from build123d import *

# Parameters (mm, degrees)
SKETCH1_R             = 40
BOSS_EXTRUDE1_DEPTH   = 105
SKETCH2_R             = 25
BOSS_EXTRUDE2_DEPTH   = 21
BOSS_EXTRUDE3_START   = 21
SKETCH3_R             = 25
BOSS_EXTRUDE3_DEPTH   = 21
FILLET1_R             = 2
SKETCH5_W             = 45.050033199
SKETCH5_H             = 42.615736352
CUT_EXTRUDE1_DEPTH    = 158.508729917
CUT_EXTRUDE2_DEPTH    = 158.508729917
SKETCH8_R             = 3.75
CUT_EXTRUDE3_DEPTH    = 158.508729917
CUT_EXTRUDE4_DEPTH    = 139.115893365
CUT_EXTRUDE5_DEPTH    = 10
FILLET2_R             = 1
BODY_MOVE_COPY1_ANGLE = 90


with BuildPart() as part:
    # Sketch1 → Boss-Extrude1 (new body)
    with BuildSketch(Plane(origin=(0, 0, 0), x_dir=(1, 0, 0), z_dir=(0, 1, 0))):
        with Locations(Location((0, 0, 0), (0, 0, 270))):
            Circle(SKETCH1_R)
    extrude(amount=BOSS_EXTRUDE1_DEPTH)

    # Sketch2 → Boss-Extrude2 (add)
    with BuildSketch(Plane(origin=(0, 105, 0), x_dir=(1, 0, 0), z_dir=(0, 1, 0))):
        with Locations(Location((0, 0, 0), (0, 0, 90))):
            Circle(SKETCH2_R)
    extrude(amount=BOSS_EXTRUDE2_DEPTH)

    # Sketch3 → Boss-Extrude3 (add)
    with BuildSketch(Plane(origin=(0, 0, 0), x_dir=(-1, 0, 0), z_dir=(0, -1, 0)).offset(BOSS_EXTRUDE3_START)):
        with Locations(Location((0, 0, 0), (0, 0, 90))):
            Circle(SKETCH3_R)
    extrude(amount=-BOSS_EXTRUDE3_DEPTH)

    # Fillet1
    fillet1_edges = [part.edges().sort_by_distance(p)[0] for p in [
        (0, 0, 25),
        (0, 105, 25),
    ]]
    fillet(fillet1_edges, radius=FILLET1_R)

    # Sketch4 → Cut-Revolve1 (revolve, cut)
    with BuildSketch(Plane(origin=(0, 0, 0), x_dir=(0, 0, -1), z_dir=(1, 0, 0)), mode=Mode.PRIVATE) as cut_revolve1_sk:
        Polygon((40, 73.5), (37.5, 71), (37.5, 34), (40, 31.5), align=None)
    revolve(cut_revolve1_sk.sketch.rotate(Axis((0, 105, 0), (0, -1, 0)), 180), axis=Axis((0, 105, 0), (0, -1, 0)), mode=Mode.SUBTRACT)

    # Sketch5 → Cut-Extrude1 (cut, through all)
    with BuildSketch(Plane(origin=(0, -21, 0), x_dir=(-1, 0, 0), z_dir=(0, -1, 0))):
        with Locations((-22.5250166, -21.307868176)):
            Rectangle(SKETCH5_W, SKETCH5_H)
    extrude(amount=-CUT_EXTRUDE1_DEPTH, mode=Mode.SUBTRACT)

    # Sketch7 → Cut-Extrude2 (cut, through all)
    with BuildSketch(Plane(origin=(0, -21, 0), x_dir=(-1, 0, 0), z_dir=(0, -1, 0))):
        with BuildLine():
            Line((12, -13), (-12, -13))
            ThreePointArc((-12, -13), (-15, -10), (-12, -7))
            Line((-12, -7), (12, -7))
            ThreePointArc((12, -7), (15, -10), (12, -13))
        make_face()
    extrude(amount=-CUT_EXTRUDE2_DEPTH, mode=Mode.SUBTRACT)

    # Sketch8 → Cut-Extrude3 (cut, through all)
    with BuildSketch(Plane(origin=(0, -21, 0), x_dir=(-1, 0, 0), z_dir=(0, -1, 0))):
        with Locations(Location((8.282209443, -30.909626441, 0), (0, 0, 270))):
            Circle(SKETCH8_R)
        with Locations((-8.282209443, -30.909626441)):
            Circle(SKETCH8_R)
        with Locations((-22.627416998, -22.627416998)):
            Circle(SKETCH8_R)
        with Locations((-30.909626441, -8.282209443)):
            Circle(SKETCH8_R)
        with Locations(Location((-30.909626441, 8.282209443, 0), (0, 0, 270))):
            Circle(SKETCH8_R)
        with Locations(Location((-22.627416998, 22.627416998, 0), (0, 0, 270))):
            Circle(SKETCH8_R)
        with Locations(Location((-8.282209443, 30.909626441, 0), (0, 0, 270))):
            Circle(SKETCH8_R)
        with Locations(Location((8.282209443, 30.909626441, 0), (0, 0, 270))):
            Circle(SKETCH8_R)
        with Locations(Location((22.627416998, 22.627416998, 0), (0, 0, 270))):
            Circle(SKETCH8_R)
        with Locations(Location((30.909626441, 8.282209443, 0), (0, 0, 270))):
            Circle(SKETCH8_R)
        with Locations(Location((30.909626441, -8.282209443, 0), (0, 0, 270))):
            Circle(SKETCH8_R)
        with Locations(Location((22.627416998, -22.627416998, 0), (0, 0, 270))):
            Circle(SKETCH8_R)
    extrude(amount=-CUT_EXTRUDE3_DEPTH, mode=Mode.SUBTRACT)

    # Sketch9 → Cut-Extrude4 (cut, through all)
    with BuildSketch(Plane.XY):
        with BuildLine():
            Line((25, 123.355095289), (40, 126))
            Line((40, 126), (30.207539179, 105))
            Line((30.207539179, 105), (40, 105))
            Line((40, 105), (40, 96))
            ThreePointArc((40, 96), (61.213203436, 104.786796564), (70, 126))
            ThreePointArc((70, 126), (40, 156), (10, 126))
            Line((10, 126), (25, 126))
            Line((25, 126), (25, 123.355095289))
        make_face()
        with BuildLine():
            Line((30.207539179, 105), (40, 126))
            Line((40, 126), (25, 123.355095289))
            Line((25, 123.355095289), (25, 107))
            ThreePointArc((25, 107), (25.585786438, 105.585786438), (27, 105))
            Line((27, 105), (30.207539179, 105))
        make_face()
        with BuildLine():
            ThreePointArc((27.321452148, 98.810766389), (16.199399791, 107.73715713), (10.45576741, 120.79055467))
            Line((10.45576741, 120.79055467), (5.531728645, 119.922313782))
            ThreePointArc((5.531728645, 119.922313782), (12.23263309, 104.693349985), (25.208360839, 94.279227454))
            Line((25.208360839, 94.279227454), (27.321452148, 98.810766389))
        make_face()
        with BuildLine():
            Line((25, 107), (25, 123.355095289))
            Line((25, 123.355095289), (10.45576741, 120.79055467))
            ThreePointArc((10.45576741, 120.79055467), (16.199399791, 107.73715713), (27.321452148, 98.810766389))
            Line((27.321452148, 98.810766389), (30.207539179, 105))
            Line((30.207539179, 105), (27, 105))
            ThreePointArc((27, 105), (25.585786438, 105.585786438), (25, 107))
        make_face()
        with BuildLine():
            Line((10.45576741, 120.79055467), (25, 123.355095289))
            Line((25, 123.355095289), (25, 126))
            Line((25, 126), (10, 126))
            ThreePointArc((10, 126), (10.114159057, 123.385327718), (10.45576741, 120.79055467))
        make_face()
        with BuildLine():
            Line((40, 105), (30.207539179, 105))
            Line((30.207539179, 105), (27.321452148, 98.810766389))
            ThreePointArc((27.321452148, 98.810766389), (33.506811582, 96.711119786), (40, 96))
            Line((40, 96), (40, 105))
        make_face()
    extrude(amount=-CUT_EXTRUDE4_DEPTH, mode=Mode.SUBTRACT)

    # Sketch10 → Cut-Extrude5 (cut)
    with BuildSketch(Plane(origin=(0, -21, 0), x_dir=(-1, 0, 0), z_dir=(0, -1, 0))):
        with BuildLine():
            Line((4, -3), (4, 4))
            Line((4, 4), (-20.615528128, 4))
            ThreePointArc((-20.615528128, 4), (3.501020872, 20.706106656), (20.784609691, -3))
            Line((20.784609691, -3), (4, -3))
        make_face()
    extrude(amount=-CUT_EXTRUDE5_DEPTH, mode=Mode.SUBTRACT)

    # Fillet2
    fillet2_edges = [part.edges().sort_by_distance(p)[0] for p in [
        (-12.392304845, -11, 3),
        (-4, -11, -0.5),
        (8.307764064, -11, -4),
        (-3.501020872, -11, -20.706106656),
    ]]
    fillet(fillet2_edges, radius=FILLET2_R)


with BuildPart() as part_1:
    # Body-Move/Copy1: moved
    add(part.part.rotate(Axis((0, 52.5, 0), (-1, 0, 0)), BODY_MOVE_COPY1_ANGLE))


solid = part_1.part
Can you work these out from the model? Positions are in its coordinate system, mm. A direction names the side the tool comes from. Give positions to 0.01 mm unless a question says otherwise; leave off trailing zeros. Use one line per item in the form item = value.
1) Will these pins go through, and if not, where does the flat tip stop? pin 1 (5 mm diameter, centred on x = -29.5, y = 22.5, fed in from -Z); pin 2 (6 mm diameter, centred on x = -22.63, y = 29.87, fed in from +Z); pin 3 (6 mm diameter, centred on x = -8.5, z = 21, fed in from -Y); pin 4 (2 mm diameter, centred on x = -24.5, z = 47.5, fed in from -Y).
Answers:
pin_1 = -52.5
pin_2 = through
pin_3 = 12.88
pin_4 = 20.13
2) If we section it at A-A (z = -36): Count the separate pieces of the cut face and the enclosed holes in it, plus the area to 3 significant figures.
Answers:
separate_pieces = 1
enclosed_holes = 9
area = 3,290 mm²
3) We'd pull the mould along Y, two halves only. Please class faces 1 (the face through (-27.491, 26.766, 18.656)), 2 (the face through (-3.6, 52.6, 73.5)), 3 (the face through (-15, 62.4, 1)): released by +Y, released by -Y, zero draft, split by the parting line, or undercut.
Answers:
face_1 = split by the parting line
face_2 = zero draft
face_3 = undercut
4) For faces 4 (the face through (-6, 65.5, 1)), 5 (the face through (-21, 35, 52.5)), 6 (the face through (-27.4, 26.9, 0.3)), which set-ups out of +Z, -Z, +X, -X, +Y, -Y let a thin tool reach every point of the face, with its end or its side?
Answers:
face_4 = +Z, -Z, +X
face_5 = +Z
face_6 = none
5) I need wall thicknesses on line 1 along Y through (x, z) = (-1, 10.5); line 2 along X through (y, z) = (18.5, 14); line 3 along X through (y, z) = (33, 24.5). Which ranges of each line are inside material? Lowest first, please.
Answers:
line_1 = 15.01 to 59.5, 65.5 to 89.99
line_2 = -15.82 to -10.41, -6.16 to 6.16, 10.41 to 15.82
line_3 = -34.92 to -24.7, -20.56 to 20.56, 24.7 to 34.92
